```python
from build123d import *

# Parameters (mm, degrees)
SKETCH2_R           = 20
BOSS_EXTRUDE1_DEPTH = 60
CUT_EXTRUDE2_DEPTH  = 50
CUT_EXTRUDE3_DEPTH  = 50
SKETCH12_W          = 16.164310213
SKETCH12_H          = 9.181328202
CUT_EXTRUDE5_DEPTH  = 40
SKETCH13_R          = 5
CUT_EXTRUDE6_DEPTH  = 40


with BuildPart() as part:
    # Sketch2 → Boss-Extrude1 (new body)
    with BuildSketch(Plane(origin=(0, 0, 0), x_dir=(0, 0, -1), z_dir=(1, 0, 0))):
        with BuildLine():
            Line((-79.56687109, 0), (-79.56687109, 10))
            Line((-79.56687109, 10), (-18.568740921, 67.473716741))
            ThreePointArc((-18.568740921, 67.473716741), (33.570555999, 62.815503761), (22.769179524, 11.595044004))
            Line((22.769179524, 11.595044004), (2.43312891, 0))
            Line((2.43312891, 0), (-79.56687109, 0))
        make_face()
        with Locations((5.43312891, 42)):
            Circle(SKETCH2_R, mode=Mode.SUBTRACT)
    extrude(amount=-BOSS_EXTRUDE1_DEPTH)


with BuildPart() as part_1:
    # Body-Move/Copy1: moved
    add(part.part.moved(Location((5, 0, 0))))

    # Sketch4 → Cut-Extrude2 (cut)
    with BuildSketch(Plane(origin=(0, 0, 0), x_dir=(0, 0, -1), z_dir=(1, 0, 0))):
        Polygon((-79.56687109, 10), (-29.56687109, 11.408616082), (-30.821121194, 55.929267243), align=None)
    extrude(amount=-CUT_EXTRUDE2_DEPTH, mode=Mode.SUBTRACT)

    # Sketch5 → Cut-Extrude3 (cut)
    with BuildSketch(Plane(origin=(0, 12.231875294, 0.344600325), x_dir=(1, 0, 0), z_dir=(0, 0.9996033962131115, 0.028161148400119476))):
        with BuildLine():
            Line((-40.497825503, -59.233865026), (-10.497825503, -59.233865026))
            ThreePointArc((-10.497825503, -59.233865026), (-5.487906474, -64.243784055), (-10.497825503, -69.253703083))
            Line((-10.497825503, -69.253703083), (-40.497825503, -69.253703083))
            ThreePointArc((-40.497825503, -69.253703083), (-45.507744532, -64.243784055), (-40.497825503, -59.233865026))
        make_face()
    extrude(amount=-CUT_EXTRUDE3_DEPTH, mode=Mode.SUBTRACT)


with BuildPart() as part_2:
    # Body-Move/Copy2: moved
    add(part_1.part.moved(Location((5, 0, 0))))

    # Sketch12 → Cut-Extrude5 (cut)
    with BuildSketch(Plane(origin=(0, 0, 0), x_dir=(0, 0, -1), z_dir=(1, 0, 0))):
        with Locations((5.433128911, 77.294344512)):
            Rectangle(SKETCH12_W, SKETCH12_H)
    extrude(amount=-CUT_EXTRUDE5_DEPTH, mode=Mode.SUBTRACT)

    # Sketch13 → Cut-Extrude6 (cut)
    with BuildSketch(Plane(origin=(0, 72.703680411, 0), x_dir=(1, 0, 0), z_dir=(0, 1, 0))):
        with Locations(Location((-21.004088917, 4.614936989, 0), (0, 0, 270))):
            Circle(SKETCH13_R)
    extrude(amount=-CUT_EXTRUDE6_DEPTH, mode=Mode.SUBTRACT)


solid = part_2.part
```
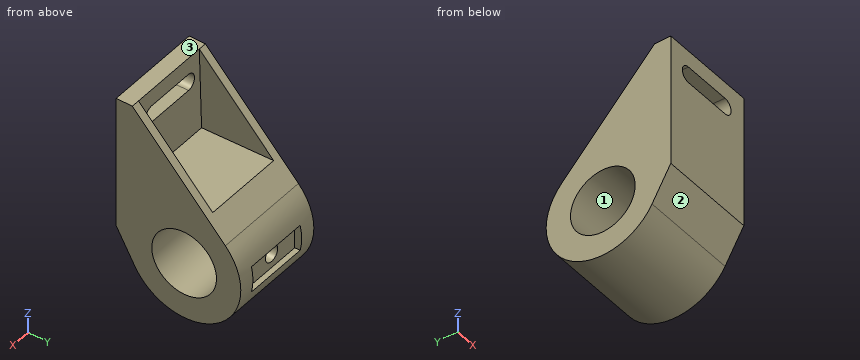
Work out the finished part from the listing and answer in its coordinate system (mm). Face numbers are marked on the shaded views. Give positions to 0.01 mm unless a question says otherwise; leave off trailing zeros. Loops run counter-clockwise (first coordinate to the right, second up) from the corner with the lowest first, then second, coordinate; pieces in that order, holes last. Notation, with made-up numbers: M 30,-12.75 L 61,-12.75 A6 ccw 61,-8.75 Z; hole C 20,51.25 d5. An arc over 180 degrees is marked long. One line per item, written item: value. Start each with the question number.
1. Find section B-B (x = 2.5). Give the vertices of the cut face in (y, z).
2. Each of these flat-tipped pins is pushed along its axis until it touches: P1, Ø1, axis at x = -39.5, y = 12, coming from the -Z side; P2, Ø18, axis at x = -27.5, z = -7, coming from the +Y side; P3, Ø1, axis at x = -10, y = 74.5, coming from the -Z side. Where does it stop, or does it pass through?
3. Find section A-A (x = -10.5). Give the vertices of the cut face in (y, z), and give its area (3 significant figures).
4. Find the intervals of material crossed by probe 1 along X at (y, z) = (32, 37); probe 2 along Y at (x, z) = (-14.5, -18); probe 3 along Z at (x, y) = (-33, 55.5), in increasing order.
5. Find section D-D (z = -19.5). Give the vertices of the cut face in (x, y), and give its area (3 significant figures).
6. Find section C-C (y = 42). Give the vertices of the cut face in (x, z), and give its area (3 significant figures).
7. Determine the mould class of the marked faces 1, 2 and 3 for opening direction Y: released by +Y, released by -Y, zero draft, split by the parting line, or undercut.
Reported:
1. outline: M 0,-2.43 L 11.6,-22.77 A35 ccw long 67.47,18.57 L 55.93,30.82 L 11.41,29.57 L 10,79.57 L 0,79.57 Z; hole C 42,-5.43 d40
2. P1: stops at z = -24.27
2. P2: stops at y = 76.05
2. P3: stops at z = -19.61
3. outline: M 0,-2.43 L 11.6,-22.77 A35 ccw 76.05,-13.52 L 72.7,-13.52 L 72.7,2.65 L 76.05,2.65 A35 ccw 67.47,18.57 L 55.93,30.82 L 11.41,29.57 L 10.56,59.55 L 0,59.26 Z; M 0,69.28 L 10.28,69.57 L 10,79.57 L 0,79.57 Z; hole C 42,-5.43 d40
3. area: 3,550 mm²
4. probe 1: x = -50 to -45, 5 to 10
4. probe 2: y = 8.88 to 26.44, 57.56 to 74.67
4. probe 3: z = -37.72 to -20.19, 9.32 to 30.81
5. outline: M -50,9.73 L 10,9.73 L 10,27.78 L -50,27.78 Z; M -50,56.22 L 10,56.22 L 10,74.05 L -50,74.05 Z
5. area: 2,150 mm²
6. outline: M -50,-40.43 L 10,-40.43 L 10,-25.43 L -50,-25.43 Z; M -50,14.57 L 10,14.57 L 10,45.6 L 5,45.6 L 5,30.43 L -45,30.43 L -45,45.6 L -50,45.6 Z
6. area: 2,000 mm²
7. face 1: undercut
7. face 2: released by -Y
7. face 3: zero draft
